from build123d import *

# Parameters (mm, degrees)
SKETCH3_R           = 4
BOSS_EXTRUDE1_DEPTH = 3


with BuildPart() as part:
    # Sketch3 → Boss-Extrude1 (new body)
    with BuildSketch(Plane(origin=(0, 0, 0), x_dir=(0, 0, -1), z_dir=(1, 0, 0))):
        with BuildLine():
            Line((-16.828358209, -0.167910448), (-16.828358209, -13.667910448))
            Line((-16.828358209, -13.667910448), (-15.328358209, -13.667910448))
            Line((-15.328358209, -13.667910448), (-15.328358209, -19.167910448))
            Line((-15.328358209, -19.167910448), (-10.328358209, -19.167910448))
            Line((-10.328358209, -19.167910448), (-10.328358209, -13.667910448))
            Line((-10.328358209, -13.667910448), (-9.078358209, -13.667910448))
            Line((-9.078358209, -13.667910448), (-9.078358209, -6.667910448))
            Line((-9.078358209, -6.667910448), (15.421641791, -6.667910448))
            Line((15.421641791, -6.667910448), (15.421641791, -13.667910448))
            Line((15.421641791, -13.667910448), (16.671641791, -13.667910448))
            Line((16.671641791, -13.667910448), (16.671641791, -19.167910448))
            Line((16.671641791, -19.167910448), (21.671641791, -19.167910448))
            Line((21.671641791, -19.167910448), (21.671641791, -13.667910448))
            Line((21.671641791, -13.667910448), (23.171641791, -13.667910448))
            Line((23.171641791, -13.667910448), (23.171641791, -0.167910448))
            ThreePointArc((23.171641791, -0.167910448), (18.726397941, 1.476700456), (16.856765964, 5.832089552))
            ThreePointArc((16.856765964, 5.832089552), (2.853872221, 19.832089253), (-11.14323284, 5.826302065))
            ThreePointArc((-11.14323284, 5.826302065), (-12.789836747, 1.694905763), (-16.828358209, -0.167910448))
        make_face()
        with Locations((2.856765964, 5.832089552)):
            Circle(SKETCH3_R, mode=Mode.SUBTRACT)
    extrude(amount=BOSS_EXTRUDE1_DEPTH)


solid = part.part
Could you check a few things on this model? Use its own coordinates, in mm. A direction names the side the tool comes from. Round coordinates to 2 decimals unless told otherwise and drop trailing zeros. Write each loop counter-clockwise with the first axis right and the second up, starting at its lowest first coordinate (ties: lowest second). Pieces come first, ordered by that corner, then holes. Notation, with made-up numbers: (-19.75, 75) - (37.25, 75) arc R19 ccw to (37.25, 101) - close; hole circle Ø8 at (11.5, 87). An arc over 180 degrees is marked (long way). Put each result on its own line as item: value. Start each with the question number.
(1) Thinking about a two-plate mould opening in Z: for faces 1 (the flat face through (1, -16, 10.328)), 2 (the cylindrical face through (1.48, 19.83, -3.16)), 3 (the flat face through (1, -13.668, -22)), which applies, released by +Z, released by -Z, zero draft, split by the parting line, or undercut?
(2) I want a section at B-B, the plane z = -5. Please give me the cut outline in (x, y), plus the area to 3 significant figures.
(3) I want a section at C-C, the plane y = 11.5. Please give me the cut outline in (x, z).
(4) I want a section at D-D, the plane z = 5.5. Please give me the cut outline in (x, y).
(5) For faces 4 (the flat face through (1, -16, 15.328)), 5 (the flat face through (1, -6.668, -3)), 6 (the flat face through (1, -16, -21.672)), which set-ups out of +Z, -Z, +X, -X, +Y, -Y let a thin tool reach every point of the face, with its end or its side?
(6) I want a section at A-A, the plane x = 0.6. Please give me the cut outline in (y, z).
(7) Will these pins go through, and if not, where does the flat tip stop? pin 1 (1 mm diameter, centred on x = 1, z = -10, fed in from -Y); pin 2 (1 mm diameter, centred on x = 2, y = 2, fed in from -Z); pin 3 (1.5 mm diameter, centred on x = 1, z = 9.5, fed in from -Y).
(8) I need wall thicknesses on probe 1 along Z at (x, y) = (2.8, -13); probe 2 along Z at (x, y) = (0.7, -16); probe 3 along Y at (x, z) = (2.9, 0.5). Which ranges of each line are inside material? Lowest first, please.
Here are the results:
1. face 1: undercut
1. face 2: split by the parting line
1. face 3: zero draft
2. outline: (0, -6.67) - (3, -6.67) - (3, 2.45) - (0, 2.45) - close; (0, 9.21) - (3, 9.21) - (3, 19.67) - (0, 19.67) - close
2. area: 58.7 mm^2
3. outline: (0, -15.66) - (3, -15.66) - (3, 9.94) - (0, 9.94) - close
4. outline: (0, -6.67) - (3, -6.67) - (3, 17.06) - (0, 17.06) - close
5. face 4: +Z, +X, -X, -Y
5. face 5: +X, -X, -Y
5. face 6: -Z, +X, -X, -Y
6. outline: (-19.17, -21.67) - (-13.67, -21.67) - (-13.67, -23.17) - (-0.17, -23.17) arc R6.01 cw to (5.83, -16.86) arc R14 ccw to (5.83, 11.14) arc R6 cw to (-0.17, 16.83) - (-13.67, 16.83) - (-13.67, 15.33) - (-19.17, 15.33) - (-19.17, 10.33) - (-13.67, 10.33) - (-13.67, 9.08) - (-6.67, 9.08) - (-6.67, -15.42) - (-13.67, -15.42) - (-13.67, -16.67) - (-19.17, -16.67) - close; hole circle Ø8 at (5.83, -2.86)
7. pin 1: stops at y = -6.67
7. pin 2: stops at z = -18.7
7. pin 3: stops at y = -13.67
8. probe 1: z = -23.17 to -15.42, 9.08 to 16.83
8. probe 2: z = -21.67 to -16.67, 10.33 to 15.33
8. probe 3: y = -6.67 to 3.66, 8.01 to 19.42
